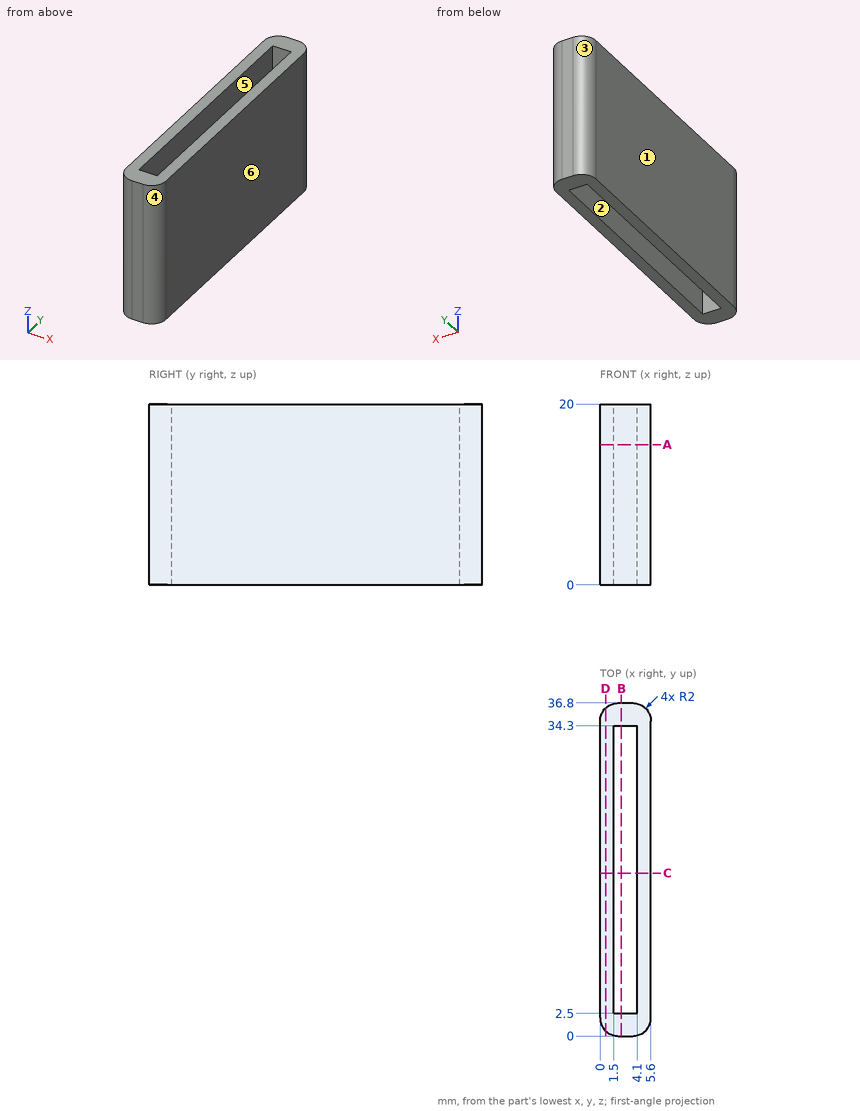
Print and shaded views of the part. All mm, measured from the part's lowest x, y and z. A direction names the side the tool comes from. Give positions to 0.01 mm unless a question says otherwise; leave off trailing zeros. Loops run counter-clockwise (first coordinate to the right, second up) from the corner with the lowest first, then second, coordinate; pieces in that order, holes last. Notation, with made-up numbers: (83.5, 18.5) - (131.5, 18.5) arc R18 ccw to (131.5, 36.5) - close; hole circle Ø8 at (-8, 40.25). An arc over 180 degrees is marked (long way). Use a Markdown table: item, result.
(1) Pull direction Y, two halves, no side cores. Call the marked faces 1, 2, 3 and 4: +Y half, -Y half, draft (parallel to the pull), parting line (faces both ways), or undercut.
Taken from the geometry:
| item | result |
|---|---|
| face 1 | draft |
| face 2 | undercut |
| face 3 | +Y half |
| face 4 | -Y half |
(2) Wall check: line 1 along X through (y, z) = (32.5, 4.5); line 2 along Y through (x, z) = (2.35, 8.75); line 3 along Y through (x, z) = (4.5, 18.25). Give the ranges that are in metal, low to high.
Taken from the geometry:
| item | result |
|---|---|
| line 1 | 0 to 1.5, 4.1 to 5.6 |
| line 2 | 0 to 2.5, 34.3 to 36.8 |
| line 3 | 0.21 to 36.59 |
(3) Band-saw the part on B-B (x = 2.35). Give the cut face in (y, z), and give its area (4 significant figures).
Taken from the geometry:
| item | result |
|---|---|
| outline | (0, 0) - (2.5, 0) - (2.5, 20) - (0, 20) - close; (34.3, 0) - (36.8, 0) - (36.8, 20) - (34.3, 20) - close |
| area | 100.0 mm2 |
(4) Band-saw the part on D-D (x = 0.6). Give the cut face in (y, z).
Taken from the geometry:
| item | result |
|---|---|
| outline | (0.57, 0) - (36.23, 0) - (36.23, 20) - (0.57, 20) - close |
(5) Band-saw the part on A-A (z = 15.5). Give the cut face in (x, y).
Taken from the geometry:
| item | result |
|---|---|
| outline | (0, 2) arc R2 ccw to (2, 0) - (3.6, 0) arc R2 ccw to (5.6, 2) - (5.6, 34.8) arc R2 ccw to (3.6, 36.8) - (2, 36.8) arc R2 ccw to (0, 34.8) - close; hole (1.5, 2.5) - (4.1, 2.5) - (4.1, 34.3) - (1.5, 34.3) - close |
(6) Band-saw the part on C-C (y = 18). Give the cut face in (x, z), and give its area (3 significant figures).
Taken from the geometry:
| item | result |
|---|---|
| outline | (0, 0) - (1.5, 0) - (1.5, 20) - (0, 20) - close; (4.1, 0) - (5.6, 0) - (5.6, 20) - (4.1, 20) - close |
| area | 60.0 mm2 |
(7) Which spindle directions (+Z, -Z, +X, -X, +Y, -Y) get a long thin tool onto all of the face, cutting with end or side? Do the marked faces 5 and 6. Say none if no direction does.
Taken from the geometry:
| item | result |
|---|---|
| face 5 | +Z, -Z |
| face 6 | +Z, -Z, +X, +Y, -Y |
